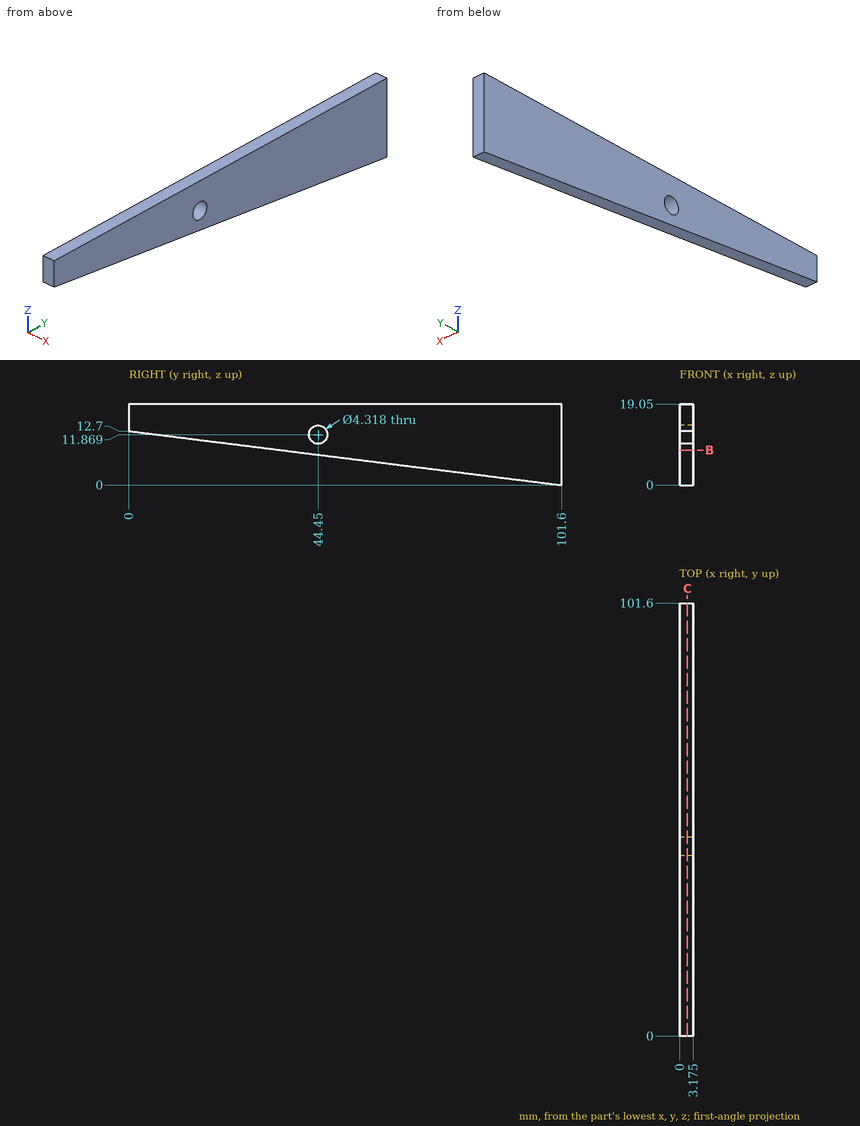
Design review of the part shown in the three views and the two pictorial views. Dimensions are in mm from the part's minimum x, y and z. Round coordinates to 2 decimals unless told otherwise and drop trailing zeros. Order: outer loops, then holes, each group sorted by start corner. A loop starts at its lowest first (then second) coordinate and runs counter-clockwise, first axis right, second up.
Q1. Insertion check: P1, Ø1, axis at x = 2, y = 21, coming from the -Z side. The pin has a flat end and moves straight along its axis. Give the tip position at first contact, or say it passes through.
Findings below:
P1: stops at z = 10.01
Q2. Wall thickness on line 1 (Z direction, x = 2.3, y = 44.45); line 2 (Z direction, x = 1.6, y = 44); line 3 (Z direction, x = 3, y = 34): over which ranges is each line inside the solid? List them lowest first.
Findings below:
line 1: z = 7.14 to 9.71, 14.03 to 19.05
line 2: z = 7.2 to 9.76, 13.98 to 19.05
line 3: z = 8.45 to 19.05
Q3. We need section C-C, the plane x = 1.8. Give the boundary of the cut face in (y, z), plus the area to 3 significant figures.
Findings below:
outline: (0, 12.7) - (101.6, 0) - (101.6, 19.05) - (0, 19.05) - close; hole circle Ø4.32 at (44.45, 11.87)
area: 1,280 mm2
Q4. We need section B-B, the plane z = 8.25. Give the boundary of the cut face in (x, y) (1 decimal).
Findings below:
outline: (0, 35.6) - (3.2, 35.6) - (3.2, 101.6) - (0, 101.6) - close
